Print and shaded views of the part. All mm, measured from the part's lowest x, y and z. Round coordinates to 2 decimals unless told otherwise and drop trailing zeros. Write each loop counter-clockwise with the first axis right and the second up, starting at its lowest first coordinate (ties: lowest second). Pieces come first, ordered by that corner, then holes. Notation, with made-up numbers: M -39.75,-17.5 L -16.75,-17.5 A23 ccw -16.75,1.5 Z; hole C 89,-8.75 d8. An arc over 180 degrees is marked long. Write item = value, one per line. Start each with the question number.
Q1. Drop flat-ended pins along their axis: P1, Ø2, axis at x = 2, y = 10, coming from the -Z side; P2, Ø1.5, axis at x = 9, z = 25.5, coming from the -Y side; P3, Ø3, axis at y = 9, z = 23.5, coming from the -X side; P4, Ø4, axis at x = 7.5, y = 1.5, coming from the -Z side. Give the stop position or say it passes through.
Q2. Band-saw the part on C-C on z = 18. Write the cut outline in (x, y).
Q3. Probe L1, parallel to X at y = 6, z = 1.6; L2, parallel to Z at x = 1.25, y = 9.5. List the from-to ranges inside material, lowest first.
Q4. Pull direction X, two halves, no side cores. Call the marked faces 1, 2 and 3: released by +X, released by -X, zero draft, split by the parting line, or undercut.
Q5. Band-saw the part on B-B on y = 6. Write the cut outline in (x, z), plus the area to 4 significant figures.
Q6. Band-saw the part on A-A on x = 6. Write the cut outline in (y, z), plus the area to 3 significant figures.
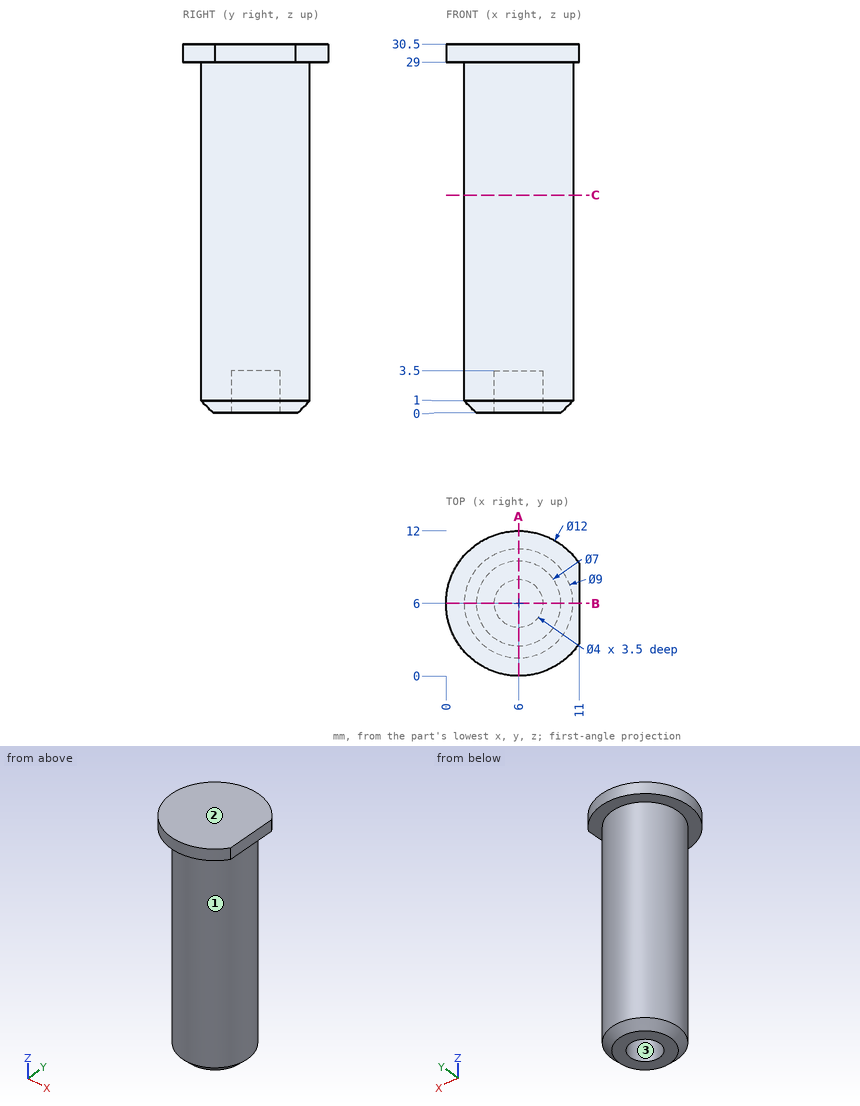
Conclusion:
q1.P1 = 29
q1.P2 = 2.1
q1.P3 = 1.76
q1.P4 = 0
q2.outline = C 6,6 d9
q3.L1 = 1.5 to 4, 8 to 10.5
q3.L2 = 29 to 30.5
q4.face_1 = split by the parting line
q4.face_2 = zero draft
q4.face_3 = undercut
q5.outline = M 0,29 L 1.5,29 L 1.5,1 L 2.5,0 L 4,0 L 4,3.5 L 8,3.5 L 8,0 L 9.5,0 L 10.5,1 L 10.5,29 L 11,29 L 11,30.5 L 0,30.5 Z
q5.area = 262.5 mm^2
q6.outline = M 0,29 L 1.5,29 L 1.5,1 L 2.5,0 L 4,0 L 4,3.5 L 8,3.5 L 8,0 L 9.5,0 L 10.5,1 L 10.5,29 L 12,29 L 12,30.5 L 0,30.5 Z
q6.area = 264 mm^2
